The figure shows three views and two pictorial views of one solid part (mm, origin at its lowest corner). Answer the questions. Give positions to 0.01 mm unless a question says otherwise; leave off trailing zeros. Order: outer loops, then holes, each group sorted by start corner. A loop starts at its lowest first (then second) coordinate and runs counter-clockwise, first axis right, second up. Notation, with made-up numbers: (5, 6.25) - (13, 6.25) arc R28 ccw to (13, 45.25) - close; hole circle Ø8 at (-23.75, 78.5). An arc over 180 degrees is marked (long way). Answer as a JSON object with one key per item and string values. Group by question number.
Q1. Consider line 1 (X direction, y = 2.2, z = 3.75) (1 decimal); line 2 (X direction, y = 1.9, z = 5.5); line 3 (Z direction, x = 10.5, y = 1.9) (1 decimal). Determine where each line is inside the solid, lowest interval first.
Q2. A cutting plane is placed at C-C, the plane z = 8. Give the vertices of the cut face in (x, y).
Q3. Given pin 1 (3.5 mm diameter, centred on x = 9.32, z = 4.5, fed in from +Y), flat-ended and moving along its own axis, determine where the tip first touches the part or whether it passes through.
Q4. A cutting plane is placed at B-B, the plane y = 1.35. Give the vertices of the cut face in (x, z).
Q5. A cutting plane is placed at A-A, the plane z = 4.5. Give the vertices of the cut face in (x, y).
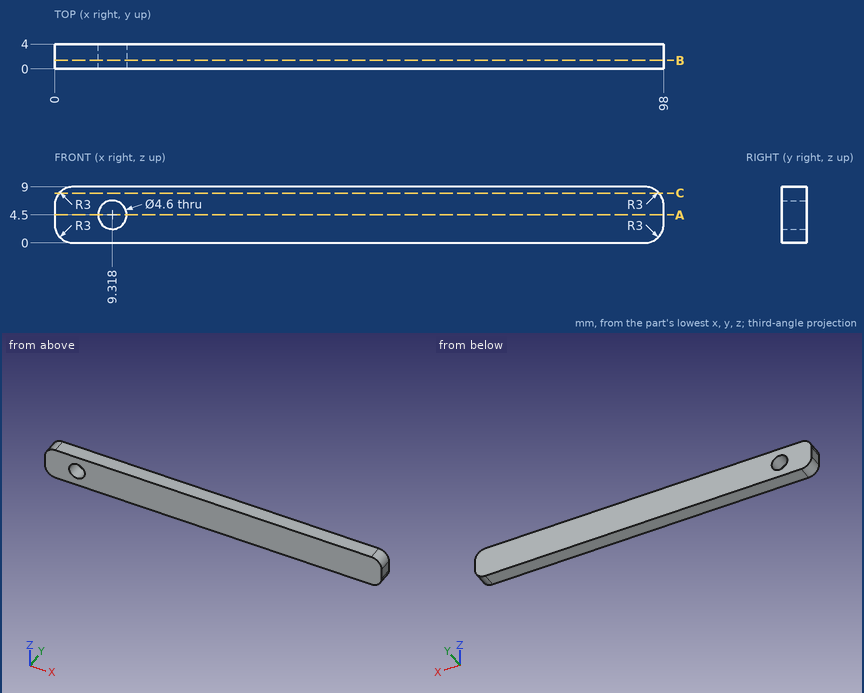
Reply:
{
 "1": {"line 1": "x = 0 to 7.1, 11.5 to 98", "line 2": "x = 0 to 7.25, 11.39 to 98", "line 3": "z = 0 to 2.5, 6.5 to 9"},
 "2": {"outline": "(0.76, 0) - (97.24, 0) - (97.24, 4) - (0.76, 4) - close"},
 "3": {"pin 1": "passes through"},
 "4": {"outline": "(0, 3) arc R3 ccw to (3, 0) - (95, 0) arc R3 ccw to (98, 3) - (98, 6) arc R3 ccw to (95, 9) - (3, 9) arc R3 ccw to (0, 6) - close; hole circle Ø4.6 at (9.32, 4.5)"},
 "5": {"outline": "(0, 0) - (7.02, 0) - (7.02, 4) - (0, 4) - close; (11.62, 0) - (98, 0) - (98, 4) - (11.62, 4) - close"}
}
